from build123d import *

# Parameters (mm, degrees)
F1_DEPTH  = 19.05
F3_DEPTH  = 12.701
F4_R      = 6.35
F5_DEPTH  = 12.701
F6_R      = 2.54
F8_DEPTH  = 76.201
F9_R      = 5.08
F11_DEPTH = 25.4


with BuildPart() as f1:
    # F0 (on Right) → F1 (new body, symmetric)
    with BuildSketch(Plane.YZ):
        Polygon((-51.152777, 0), (0, 0), (25.047223, 0), (25.047223, 38.1), (12.347223, 38.1), (12.347223, 12.7), (-51.152777, 12.7), align=None)
    extrude(amount=F1_DEPTH, both=True)

    # F2 (on face) → F3 (cut, through all)
    with BuildSketch(Plane.XZ.offset(-12.347223)):
        with BuildLine():
            ThreePointArc((-8.801841, 30.474761), (0, 35.56), (8.801841, 30.474761))
            Line((8.801841, 30.474761), (19.05, 12.7))
            Line((19.05, 12.7), (19.05, 38.1))
            Line((19.05, 38.1), (-19.05, 38.1))
            Line((-19.05, 38.1), (-19.05, 12.7))
            Line((-19.05, 12.7), (-8.801841, 30.474761))
        make_face()
    extrude(amount=-F3_DEPTH, mode=Mode.SUBTRACT)

    # F4 (on face) → F5 (cut, through all)
    with BuildSketch(Plane.XZ.offset(-12.347223)):
        with Locations((0, 25.4)):
            Circle(F4_R)
    extrude(amount=-F5_DEPTH, mode=Mode.SUBTRACT)

    # F6
    f6_edges = [f1.edges().sort_by_distance(p)[0] for p in [
        (0, 12.347223, 12.7),
    ]]
    fillet(f6_edges, radius=F6_R)

    # F7 (on face) → F8 (cut, through all)
    with BuildSketch(Plane.XZ.offset(51.152777)):
        Polygon((-6.35, 0), (0, 0), (6.35, 0), (6.35, 2.49879), (11.43, 2.49879), (11.43, 4.806255), (-11.43, 4.806255), (-11.43, 2.266255), (-6.35, 2.266255), align=None)
    extrude(amount=-F8_DEPTH, mode=Mode.SUBTRACT)

    # F9
    f9_edges = [f1.edges().sort_by_distance(p)[0] for p in [
        (0, -51.152777, 12.7),
    ]]
    fillet(f9_edges, radius=F9_R)

    # F10 (on face) → F11 (cut)
    with BuildSketch(Plane.XY.offset(12.7)):
        with BuildLine():
            Line((3.80817, -16.744703), (3.808204, -16.979764))
            ThreePointArc((3.808204, -16.979764), (3.81, -16.862233), (3.80817, -16.744703))
        make_face()
        with BuildLine():
            Line((3.81, -29.562233), (3.808204, -16.979764))
            Line((3.808204, -16.979764), (3.80817, -16.744703))
            ThreePointArc((3.80817, -16.744703), (-0.018418, -13.052821), (-3.809134, -16.781525))
            Line((-3.809134, -16.781525), (-3.809144, -16.943512))
            Line((-3.809144, -16.943512), (-3.81, -29.562519))
            ThreePointArc((-3.81, -29.562519), (0.000143, -33.372777), (3.81, -29.562233))
        make_face()
        with BuildLine():
            Line((-3.809144, -16.943512), (-3.809134, -16.781525))
            ThreePointArc((-3.809134, -16.781525), (-3.81, -16.862519), (-3.809144, -16.943512))
        make_face()
    extrude(amount=-F11_DEPTH, mode=Mode.SUBTRACT)


solid = f1.part
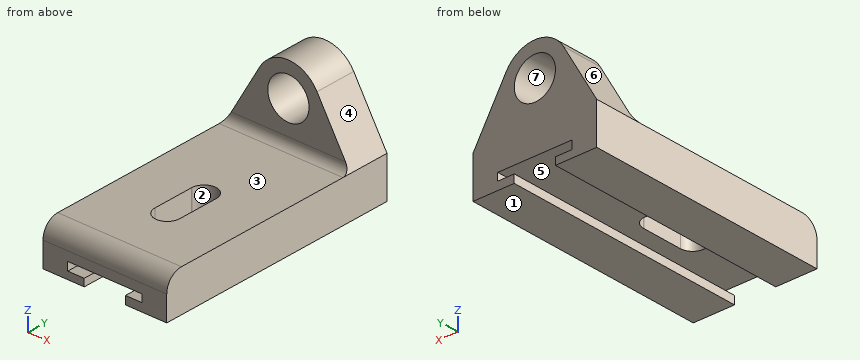
Geometry check sheet. Reference: the model listing, model coordinates, mm. Face numbers are marked on the shaded views. A direction names the side the tool comes from. Round coordinates to 2 decimals unless told otherwise and drop trailing zeros. Loops run counter-clockwise (first coordinate to the right, second up) from the corner with the lowest first, then second, coordinate; pieces in that order, holes last.
Item 1: Mould release check, pull along X, two halves, no side actions. Record for the marked faces 4, 5, 6 and 7: pulls with the +X half, pulls with the -X half, needs draft (parallel to the pull), parting line crosses it, or undercut.
Item 2: Cross-section at B-B on y = 19. Record the boundary of the cut face in (x, z), then the cut area to 3 significant figures.
Item 3: Cross-section at D-D on z = 25.4. Record the boundary of the cut face in (x, y), then the cut area to 3 significant figures.
Item 4: Cross-section at A-A on x = 0. Record the boundary of the cut face in (y, z).
Item 5: Thickness scan on line 1 (Z direction, x = 9, y = -8.5); line 2 (Z direction, x = 0, y = 17); line 3 (Z direction, x = 3, y = 5.5). Record the ranges inside material, lowest first.
Item 6: Gauge pin test, flat ends, axial feed: pin 1 (11.5 mm diameter, centred on x = 0, z = 25.4, fed in from -Y); pin 2 (8 mm diameter, centred on x = -3.5, y = -30, fed in from +Z); pin 3 (7 mm diameter, centred on x = -2.5, y = -22.5, fed in from -Z); pin 4 (16.5 mm diameter, centred on x = 8.5, z = 27.5, fed in from -Y). Record the tip position at first contact, or that the pin passes through.
Item 7: Access from +Z, -Z, +X, -X, +Y, -Y to the whole of each face (thin tool, end or side, straight path). Record for the marked faces 1, 2 and 3.
Item 8: Cross-section at C-C on y = -21. Record the boundary of the cut face in (x, z).
Answer sheet:
1. face 4: pulls with the +X half
1. face 5: undercut
1. face 6: pulls with the -X half
1. face 7: undercut
2. outline: (-19.05, 0) - (-6.35, 0) - (-6.35, 2.27) - (-11.43, 2.27) - (-11.43, 4.81) - (11.43, 4.81) - (11.43, 2.5) - (6.35, 2.5) - (6.35, 0) - (19.05, 0) - (19.05, 12.7) - (8.8, 30.47) arc R10.16 ccw to (-8.8, 30.47) - (-19.05, 12.7) - close; hole circle Ø12.7 at (0, 25.4)
2. area: 830 mm2
3. outline: (-11.73, 12.35) - (-6.35, 12.35) - (-6.35, 25.05) - (-11.73, 25.05) - close; (6.35, 12.35) - (11.73, 12.35) - (11.73, 25.05) - (6.35, 25.05) - close
3. area: 137 mm2
4. outline: (-51.15, 4.81) - (-33.37, 4.81) - (-33.37, 12.7) - (-46.07, 12.7) arc R5.08 ccw to (-51.15, 7.62) - close; (-13.05, 4.81) - (25.05, 4.81) - (25.05, 19.05) - (12.35, 19.05) - (12.35, 15.24) arc R2.54 cw to (9.81, 12.7) - (-13.05, 12.7) - close; (12.35, 31.75) - (25.05, 31.75) - (25.05, 35.56) - (12.35, 35.56) - close
5. line 1: z = 0 to 2.5, 4.81 to 12.7
5. line 2: z = 4.81 to 19.05, 31.75 to 35.56
5. line 3: z = 4.81 to 12.7
6. pin 1: passes through
6. pin 2: stops at z = 12.7
6. pin 3: stops at z = 4.81
6. pin 4: stops at y = 12.35
7. face 1: -Z, +X, -X, +Y, -Y
7. face 2: +Z, -Z
7. face 3: +Z, +X, -X, -Y
8. outline: (-19.05, 0) - (-6.35, 0) - (-6.35, 2.27) - (-11.43, 2.27) - (-11.43, 4.81) - (-3.81, 4.81) - (-3.81, 12.7) - (-19.05, 12.7) - close; (3.81, 4.81) - (11.43, 4.81) - (11.43, 2.5) - (6.35, 2.5) - (6.35, 0) - (19.05, 0) - (19.05, 12.7) - (3.81, 12.7) - close
